```python
from build123d import *

# Parameters (mm, degrees)
SKETCH1_W               = 8
SKETCH1_H               = 8
BOSS_EXTRUDE1_DEPTH     = 3
CUT_EXTRUDE1_DEPTH      = 12.704699911
CUT_EXTRUDE1_DEPTH_BACK = 12.704699911
CUT_EXTRUDE2_DEPTH      = 11
SKETCH4_R               = 1.8
CUT_EXTRUDE3_DEPTH      = 0.8
SKETCH5_W               = 8
SKETCH5_H               = 1
BOSS_EXTRUDE2_DEPTH     = 2
FILLET1_R               = 4
SKETCH6_W               = 0.961538461
SKETCH6_H               = 0.961538462
CUT_EXTRUDE4_DEPTH      = 0.4


with BuildPart() as part:
    # Sketch1 → Boss-Extrude1 (new body)
    with BuildSketch(Plane(origin=(0, 0, 0), x_dir=(1, 0, 0), z_dir=(0, 1, 0))):
        with Locations((4, 4)):
            Rectangle(SKETCH1_W, SKETCH1_H)
    extrude(amount=BOSS_EXTRUDE1_DEPTH)

    # Sketch2 → Cut-Extrude1 (cut, two sides: drawn at the far end of the back side and taken through both)
    with BuildSketch(Plane.XY.offset(-CUT_EXTRUDE1_DEPTH_BACK)):
        Polygon((0, 0), (0.6, 3), (0, 3), align=None)
        Polygon((8, 0), (7.4, 3), (8, 3), align=None)
    extrude(amount=CUT_EXTRUDE1_DEPTH + CUT_EXTRUDE1_DEPTH_BACK, mode=Mode.SUBTRACT)

    # Sketch3 → Cut-Extrude2 (cut)
    with BuildSketch(Plane(origin=(0, 0, 0), x_dir=(0, 0, -1), z_dir=(1, 0, 0))):
        Polygon((0, 0), (0.6, 3), (0, 3), align=None)
        Polygon((8, 3), (7.4, 3), (8, 0), align=None)
    extrude(amount=CUT_EXTRUDE2_DEPTH, mode=Mode.SUBTRACT)

    # Sketch4 → Cut-Extrude3 (cut)
    with BuildSketch(Plane.XZ):
        with Locations(Location((4, -3.75, 0), (0, 0, 270))):
            Circle(SKETCH4_R)
    extrude(amount=-CUT_EXTRUDE3_DEPTH, mode=Mode.SUBTRACT)

    # Sketch5 → Boss-Extrude2 (add)
    with BuildSketch(Plane.XZ):
        with Locations((4, -7.5)):
            Rectangle(SKETCH5_W, SKETCH5_H)
    extrude(amount=BOSS_EXTRUDE2_DEPTH)

    # Fillet1
    # the kernel refuses this fillet: 4 mm, written as the material it takes off along each edge
    with BuildSketch(Plane(origin=(8, -2, -16.660254038), x_dir=(0, 1, 0), z_dir=(0, 0, 1)), Plane(origin=(0, -2, 1.660254038), x_dir=(0, 1, 0), z_dir=(0, 0, -1))) as fillet1_piece_1:
        with BuildLine():
            CenterArc((4, 3.464101615), FILLET1_R, 180, 60)
            Line((0, 3.464101615), (-0.08, 3.464101615))
            Line((-0.08, 3.464101615), (-0.08, 0))
            Line((-0.08, 0), (0, -0.08))
            ThreePointArc((0, -0.08), (1, -0.08), (1.96, -0.069282032))
            Line((1.96, -0.069282032), (2, 0))
        make_face()
    extrude(amount=18.320508076, mode=Mode.SUBTRACT)

    # Sketch6 → Cut-Extrude4 (cut)
    with BuildSketch(Plane(origin=(0, 3, 0), x_dir=(1, 0, 0), z_dir=(0, 1, 0))):
        with Locations((4.106375193, 5.877622732)):
            Rectangle(SKETCH6_W, SKETCH6_H)
        with BuildLine():
            Line((3.625605963, 3.666084271), (4.587144424, 3.666084271))
            Line((4.587144424, 3.666084271), (4.587144424, 2.966965681))
            add(Edge.make_bspline(
                [(4.587144424, 2.966965681), (4.586700802, 2.899821455), (4.585863185, 2.773044347), (4.571180714, 2.594207821), (4.550779556, 2.437158718), (4.518324342, 2.299878361), (4.47486997, 2.175902827), (4.413432502, 2.062461013), (4.337876173, 1.953901165), (4.245458326, 1.85350819), (4.139144335, 1.760654771), (4.017702284, 1.679908688), (3.88401418, 1.607967915), (3.787969656, 1.570094118), (3.738787052, 1.550699655)],
                knots=[0, 0, 0, 0, 1.347156832, 2.543608823, 3.599300285, 4.522475688, 5.370350604, 6.227678973, 7.103274953, 8.018757603, 8.959280198, 9.929437417, 10.939703653, 12, 12, 12, 12], degree=3))
            Line((3.738787052, 1.550699655), (3.561503399, 1.93531504))
            add(Edge.make_bspline(
                [(3.561503399, 1.93531504), (3.604439047, 1.952873279), (3.686527672, 1.986442858), (3.795938691, 2.052543314), (3.885105421, 2.129792439), (3.955780801, 2.218165676), (4.006656804, 2.32038588), (4.045456087, 2.435104657), (4.0674697, 2.56519407), (4.07197182, 2.656725854), (4.074323911, 2.704545809)],
                knots=[0, 0, 0, 0, 1.115416734, 2.132564161, 3.06091458, 3.941973359, 4.836922823, 5.794989041, 6.848011894, 8, 8, 8, 8], degree=3))
            Line((4.074323911, 2.704545809), (3.625605963, 2.704545809))
            Line((3.625605963, 2.704545809), (3.625605963, 3.666084271))
        make_face()
    extrude(amount=-CUT_EXTRUDE4_DEPTH, mode=Mode.SUBTRACT)


solid = part.part
```
Verification items for the finished model (mm, model axes). A direction names the side the tool comes from. Give positions to 0.01 mm unless a question says otherwise; leave off trailing zeros. Loops run counter-clockwise (first coordinate to the right, second up) from the corner with the lowest first, then second, coordinate; pieces in that order, holes last.
1. Section check B-B, the plane z = -6. Enter the section's corners in (x, y).
2. Section check A-A, the plane y = 0.2. Enter the section's corners in (x, z).
3. Go/stop test with flat-tipped pins: pin 1 Ø2 at (x, y) = (1.5, -1.5) entering from +Z; pin 2 Ø2 at (x, z) = (3.5, -4.5) entering from -Y; pin 3 Ø0.8 at (x, z) = (4, -5.5) entering from +Y; pin 4 Ø2 at (y, z) = (2.5, -5.5) entering from -X. Record where each tip stops, or that it passes through.
4. Section check D-D, the plane z = -4.75. Enter the section's corners in (x, y), then the cut area to 3 significant figures.
5. Thickness scan on line 1 (Y direction, x = 6, z = -3.5); line 2 (Y direction, x = 4.25, z = -2); line 3 (Z direction, x = 7.75, y = -0.3). Record the ranges inside material, lowest first.
6. Set-up check for faces 5 (the flat face through (4, 2.6, -6)), 6 (the flat face through (4, -1, -7)), 7 (the cylindrical face through (4.541, 0.394, -5.467)): record each of +Z, -Z, +X, -X, +Y, -Y from which the full face is reachable in a straight line by a thin tool's end or side.
7. Mould release check, pull along X, two halves, no side actions. Record for faces 1 (the flat face through (4, 0.8, -4)), 2 (the flat face through (7.7, 1.5, -4.1)), 3 (the flat face through (4, -1, -8)), 4 (the flat face through (0.3, 1.5, -4.1)): released by +X, released by -X, zero draft, split by the parting line, or undercut.
8. Section check C-C, the plane x = 1.75. Enter the section's corners in (y, z), then the cut area to 3 significant figures.
Geometry says:
1. outline: (0, 0) - (8, 0) - (7.4, 3) - (4.59, 3) - (4.59, 2.6) - (3.63, 2.6) - (3.63, 3) - (0.6, 3) - close
2. outline: (0.04, -7.96) - (7.96, -7.96) - (7.96, -0.04) - (0.04, -0.04) - close; hole circle Ø3.6 at (4, -3.75)
3. pin 1: stops at z = -7
3. pin 2: stops at y = 0
3. pin 3: stops at y = 3
3. pin 4: stops at x = 0.3
4. outline: (0, 0) - (2.5, 0) - (2.5, 0.8) - (5.5, 0.8) - (5.5, 0) - (8, 0) - (7.4, 3) - (0.6, 3) - close
4. area: 19.8 mm2
5. line 1: y = 0 to 3
5. line 2: y = 0.8 to 2.6
5. line 3: z = -8 to -7
6. face 5: +Y
6. face 6: +Z, +X, -X, -Y
6. face 7: -Y
7. face 1: undercut
7. face 2: released by +X
7. face 3: zero draft
7. face 4: released by -X
8. outline: (-1.61, -8) - (0, -8) - (3, -7.4) - (3, -0.6) - (0, 0) - (0, -7) - (-1.61, -7) - close
8. area: 23.8 mm2
